```python
from build123d import *

# Parameters (mm, degrees)
F0_W      = 50
F0_H      = 22
F1_DEPTH  = 5
F2_W      = 25
F2_H      = 25
F3_DEPTH  = 7
F4_R      = 6
F5_DEPTH  = 25
F6_R      = 4
F7_DEPTH  = 34
F8_R      = 2
F9_DEPTH  = 10
F10_R     = 2.5
F11_DEPTH = 25
F12_W     = 6
F12_H     = 6
F13_DEPTH = 10


with BuildPart() as f1:
    # F0 (on Top) → F1 (new body, symmetric)
    with BuildSketch(Plane.XY):
        with Locations((-25, 23.3168965802)):
            Rectangle(F0_W, F0_H)
        Polygon((-50, 12.3168965802), (-50, 34.3168965802), (-87, 22.3168965802), (-87, 12.3168965802), align=None)
        Polygon((22, 12.3168965802), (0, 34.3168965802), (0, 12.3168965802), align=None)
        with BuildLine():
            Line((22, 12.3168965802), (0, 12.3168965802))
            ThreePointArc((0, 12.3168965802), (8.709361095, 8.709361095), (12.3168965802, 0))
            Line((12.3168965802, 0), (22, 0))
            Line((22, 0), (22, 12.3168965802))
        make_face()
        with BuildLine():
            Line((22, 0), (12.3168965802, 0))
            ThreePointArc((12.3168965802, 0), (8.709361095, -8.709361095), (0, -12.3168965802))
            Line((0, -12.3168965802), (22, -12.3168965802))
            Line((22, -12.3168965802), (22, 0))
        make_face()
        Polygon((22, -12.3168965802), (0, -12.3168965802), (-50, -12.3168965802), (-87, -12.3168965802), (-87, -22.3168965802), (-50, -34.3168965802), (0, -34.3168965802), align=None)
    extrude(amount=F1_DEPTH, both=True)

    # F2 (on face) → F3 (join)
    with BuildSketch(Plane.YZ.offset(22)):
        Rectangle(F2_W, F2_H)
    extrude(amount=-F3_DEPTH)

    # F4 (on face) → F5 (join)
    with BuildSketch(Plane.YZ.offset(22)):
        Circle(F4_R)
    extrude(amount=F5_DEPTH)

    # F6 (on face) → F7 (join)
    with BuildSketch(Plane.YZ.offset(22)):
        with Locations((8, 8)):
            Circle(F6_R)
        with Locations((-8, 8)):
            Circle(F6_R)
        with Locations((8, -8)):
            Circle(F6_R)
        with Locations((-8, -8)):
            Circle(F6_R)
    extrude(amount=F7_DEPTH)

    # F8 (on face) → F9 (cut)
    with BuildSketch(Plane.YZ.offset(56)):
        with Locations((8, 8)):
            Circle(F8_R)
        with Locations((-8, 8)):
            Circle(F8_R)
        with Locations((8, -8)):
            Circle(F8_R)
        with Locations((-8, -8)):
            Circle(F8_R)
    extrude(amount=-F9_DEPTH, mode=Mode.SUBTRACT)

    # F10 (on face) → F11 (join)
    with BuildSketch(Plane(origin=(15, 0, 0), x_dir=(0, -1, 0), z_dir=(-1, 0, 0))):
        Circle(F10_R)
    extrude(amount=F11_DEPTH)

    # F12 (on Front) → F13 (join)
    with BuildSketch(Plane.XZ):
        with Locations((44, 0)):
            Rectangle(F12_W, F12_H)
    extrude(amount=F13_DEPTH)


solid = f1.part
```
Verification items for the finished model (mm, model axes). A direction names the side the tool comes from. Give positions to 0.01 mm unless a question says otherwise; leave off trailing zeros. Order: outer loops, then holes, each group sorted by start corner. A loop starts at its lowest first (then second) coordinate and runs counter-clockwise, first axis right, second up. Notation, with made-up numbers: (69, -5) -> (125, -5) arc R26 ccw to (125, 19) -> close; hole circle Ø7 at (39, 14). An arc over 180 degrees is marked (long way). One line per item, written item: value.
(1) Sectioned sample at D-D on x = 5. Record the cut outline in (y, z).
Final values:
outline: (-29.32, -5) -> (-11.26, -5) -> (-11.26, 5) -> (-29.32, 5) -> close; circle Ø5 at (0, 0); (11.26, -5) -> (29.32, -5) -> (29.32, 5) -> (11.26, 5) -> close
(2) Sectioned sample at B-B on z = -8. Record the cut outline in (x, y).
Final values:
outline: (15, -12.5) -> (22, -12.5) -> (22, -12) -> (56, -12) -> (56, -10) -> (46, -10) -> (46, -6) -> (56, -6) -> (56, -4) -> (22, -4) -> (22, 4) -> (56, 4) -> (56, 6) -> (46, 6) -> (46, 10) -> (56, 10) -> (56, 12) -> (22, 12) -> (22, 12.5) -> (15, 12.5) -> close
(3) Scan lines: line 1 along Z through (x, y) = (50, 8); line 2 along Y through (x, z) = (-40, -3.25); line 3 along Z through (x, y) = (-54, 13). Record each from-to range of solid material in increasing order. Write a range as [from, to].
Final values:
line 1: [-12, -10], [-6, -4], [4, 6], [10, 12]
line 2: [-34.32, -12.32], [12.32, 34.32]
line 3: [-5, 5]
(4) Tool access check on faces 4 (the face through (38.8, 4.8, -10.4)), 5 (the face through (-43, -12.317, 0)), 6 (the face through (15, 0, -9)). Record the directions out of +Z, -Z, +X, -X, +Y, -Y that give a thin tool (end or side, any length) a straight path to the whole face; none if there is none.
Final values:
face 4: +X
face 5: +Z, -Z, -X
face 6: -Z, -X, +Y, -Y
(5) Sectioned sample at C-C on y = -8. Record the cut outline in (x, z).
Final values:
outline: (9.37, -5) -> (15, -5) -> (15, -12.5) -> (22, -12.5) -> (22, -12) -> (56, -12) -> (56, -10) -> (46, -10) -> (46, -6) -> (56, -6) -> (56, -4) -> (22, -4) -> (22, 4) -> (56, 4) -> (56, 6) -> (46, 6) -> (46, 10) -> (56, 10) -> (56, 12) -> (22, 12) -> (22, 12.5) -> (15, 12.5) -> (15, 5) -> (9.37, 5) -> close; (41, -3) -> (47, -3) -> (47, 3) -> (41, 3) -> close
(6) Sectioned sample at A-A on x = -38. Record the cut outline in (y, z), then the cut area to 3 significant figures.
Final values:
outline: (-34.32, -5) -> (-12.32, -5) -> (-12.32, 5) -> (-34.32, 5) -> close; (12.32, -5) -> (34.32, -5) -> (34.32, 5) -> (12.32, 5) -> close
area: 440 mm^2
(7) Gauge pin test, flat ends, axial feed: pin 1 (1.2 mm diameter, centred on y = 8, z = 8.5, fed in from +X); pin 2 (12.5 mm diameter, centred on y = 0, z = -2, fed in from +X); pin 3 (2 mm diameter, centred on x = 17, z = -2, fed in from -Y); pin 4 (2 mm diameter, centred on y = 1, z = 7.5, fed in from -X). Record the tip position at first contact, or that the pin passes through.
Final values:
pin 1: x = 46
pin 2: x = 56
pin 3: y = -18.32
pin 4: x = 15
(8) Draft check along Z on faces 1 (the face through (19, 0, -12.5)), 2 (the face through (38.8, -11.2, 5.6)), 3 (the face through (18.5, -12.5, 5.4)). Enter one of: pulls with the +Z half, pulls with the -Z half, needs draft (parallel to the pull), parting line crosses it, or undercut.
Final values:
face 1: pulls with the -Z half
face 2: undercut
face 3: needs draft
